Source: CAD feature listing. Evaluate the final solid. Frame: model axes, mm. A direction names the side the tool comes from. Give positions to 0.01 mm unless a question says otherwise; leave off trailing zeros. Order: outer loops, then holes, each group sorted by start corner. A loop starts at its lowest first (then second) coordinate and runs counter-clockwise, first axis right, second up. Notation, with made-up numbers: (13.25, -11.5) -> (19.25, -11.5) arc R8 ccw to (19.25, -2.5) -> close; hole circle Ø4 at (26.5, 6). An arc over 180 degrees is marked (long way). Use CSV: the item, a comma, the result in double quotes.
```python
from build123d import *

# Parameters (mm, degrees)
BOSS_EXTRUDE1_DEPTH = 44
SKETCH2_R           = 10
CUT_EXTRUDE1_DEPTH  = 73.707908786
SKETCH3_W           = 20
SKETCH3_H           = 20
CUT_EXTRUDE2_DEPTH  = 87.977008456
RIB3_REACH          = 63.923
SKETCH4_WALL_W      = 168.272117334
SKETCH4_WALL_H      = 10


with BuildPart() as part:
    # Sketch1 → Boss-Extrude1 (new body)
    with BuildSketch(Plane(origin=(0, 0, 0), x_dir=(0, 0, -1), z_dir=(1, 0, 0))):
        Polygon((-18.8, -7), (-18.8, -27), (51.2, -27), (51.2, 23), (11.2, 23), (11.2, -7), align=None)
    extrude(amount=BOSS_EXTRUDE1_DEPTH)

    # Sketch2 → Cut-Extrude1 (cut, through all)
    with BuildSketch(Plane(origin=(44, 0, 0), x_dir=(0, 0, -1), z_dir=(1, 0, 0))):
        with Locations((31.2, 23)):
            Circle(SKETCH2_R)
    extrude(amount=-CUT_EXTRUDE1_DEPTH, mode=Mode.SUBTRACT)

    # Sketch3 → Cut-Extrude2 (cut, through all)
    with BuildSketch(Plane.XY.offset(18.8)):
        with Locations((22, -27)):
            Rectangle(SKETCH3_W, SKETCH3_H)
    extrude(amount=-CUT_EXTRUDE2_DEPTH, mode=Mode.SUBTRACT)

    # Sketch4 wall → Rib3 (add, up to next)
    with BuildSketch(Plane(origin=(22, 8, 3.8), x_dir=(0, -0.707106781187, 0.707106781187), z_dir=(0, -0.707106781187, -0.707106781187)), mode=Mode.PRIVATE) as rib3_sk1:
        Rectangle(SKETCH4_WALL_W, SKETCH4_WALL_H)
    rib3_tool1 = extrude(rib3_sk1.sketch, amount=RIB3_REACH, mode=Mode.PRIVATE) - part.part
    add(rib3_tool1.solids().sort_by_distance((22, 8, 3.8))[0])


solid = part.part
```
1. Ray query, line 1 along X through (y, z) = (-19.5, -4); line 2 along Y through (x, z) = (27.5, 13.5); line 3 along Z through (x, y) = (40, 11.5). Return the intervals inside material, ascending.
Answer below:
line 1,"x = 0 to 12, 32 to 44"
line 2,"y = -17 to -7"
line 3,"z = -51.2 to -11.2"
2. Section query B-B on y = -2. Return loops of the section in (x, z).
Answer below:
outline,"(0, -51.2) -> (44, -51.2) -> (44, -11.2) -> (27, -11.2) -> (27, 13.8) -> (17, 13.8) -> (17, -11.2) -> (0, -11.2) -> close"
3. Section query A-A on z = -13. Return loops of the section in (x, y).
Answer below:
outline,"(0, -27) -> (12, -27) -> (12, -17) -> (32, -17) -> (32, -27) -> (44, -27) -> (44, 23) -> (0, 23) -> close"
4. Mould query, pull axis X, two halves, no side actions, for faces 1 (the flat face through (35, 8, -11.2)), 2 (the flat face through (0, -7, -23)), 3 (the flat face through (32, -22, -16)). Classes: released by +X, released by -X, zero draft, split by the parting line, or undercut.
Answer below:
face 1,"zero draft"
face 2,"released by -X"
face 3,"undercut"
5. Access query for faces 4 (the flat face through (8, 8, -11.2)), 5 (the flat face through (35, -7, 4)), 6 (the flat face through (22, -17, -16)), 7 (the cylindrical face through (22, 13, -31)). Directions: +Z, -Z, +X, -X, +Y, -Y. A direction counts if a zero-diameter tool reaches every point of the face in a straight line with its end or side. Return the directions, or none.
Answer below:
face 4,"+Z, -X, +Y"
face 5,"+Z, +X, +Y"
face 6,"+Z, -Z, -Y"
face 7,"+X, -X, +Y"
6. Section query C-C on z = 4.5. Return loops of the section in (x, y), plus the area to 3 significant figures.
Answer below:
outline,"(0, -27) -> (12, -27) -> (12, -17) -> (32, -17) -> (32, -27) -> (44, -27) -> (44, -7) -> (27, -7) -> (27, 7.3) -> (17, 7.3) -> (17, -7) -> (0, -7) -> close"
area,"823 mm²"
7. Pin query (flat end, axial travel): P1, Ø5, axis at x = 35, z = -3, coming from the +Y side; P2, Ø4, axis at y = 10, z = -3, coming from the +X side; P3, Ø5, axis at x = 34, y = 9, coming from the +Z side. Return the tip coordinate at first contact, or that it passes through.
Answer below:
P1,"stops at y = -7"
P2,"stops at x = 27"
P3,"stops at z = -11.2"
8. Section query D-D on z = -6. Return loops of the section in (x, y).
Answer below:
outline,"(0, -27) -> (12, -27) -> (12, -17) -> (32, -17) -> (32, -27) -> (44, -27) -> (44, -7) -> (27, -7) -> (27, 17.8) -> (17, 17.8) -> (17, -7) -> (0, -7) -> close"
